Build history of the part. All positions in model axes, mm. Face numbers are marked on the shaded views. Give positions to 0.01 mm unless a question says otherwise; leave off trailing zeros. Write each loop counter-clockwise with the first axis right and the second up, starting at its lowest first coordinate (ties: lowest second). Pieces come first, ordered by that corner, then holes. Notation, with made-up numbers: (-15.75, 24.5) -> (-7.75, 24.5) arc R23 ccw to (-7.75, 45.5) -> close; hole circle Ø7 at (-4.75, 19). An arc over 180 degrees is marked (long way). Put each result on its own line as item: value. Start each with the question number.
Item 1: Slice it at A-A, the plane y = 0. List the corners of the cut face in (x, z), plus the area to 3 significant figures.
Item 2: Flat gauge pins, fed straight in: pin 1 Ø6 at (x, y) = (14.5, 7.5) entering from -Z; pin 2 Ø6 at (x, y) = (31, 19.5) entering from +Z; pin 3 Ø3 at (x, z) = (26, 6) entering from +Y. Where does each tip first touch, or does it go through?
Item 3: Drill centre lines: line 1 along X through (y, z) = (30.75, 0); line 2 along Z through (x, y) = (12.75, 0); line 3 along Z through (x, y) = (38, -16). Where is each one in solid material? Low to high.
Item 4: Two-plate mould, pull along Y, no slides. Class the marked faces 1, 2 and 3: pulls with the +Y half, pulls with the -Y half, needs draft (parallel to the pull), parting line crosses it, or undercut.
Item 5: Slice it at D-D, the plane x = 16. List the corners of the cut face in (y, z), plus the area to 3 significant figures.
Item 6: Slice it at C-C, the plane z = 0. Give the number of separate pieces and of enclosed holes in the cut face, plus the area to 3 significant figures.
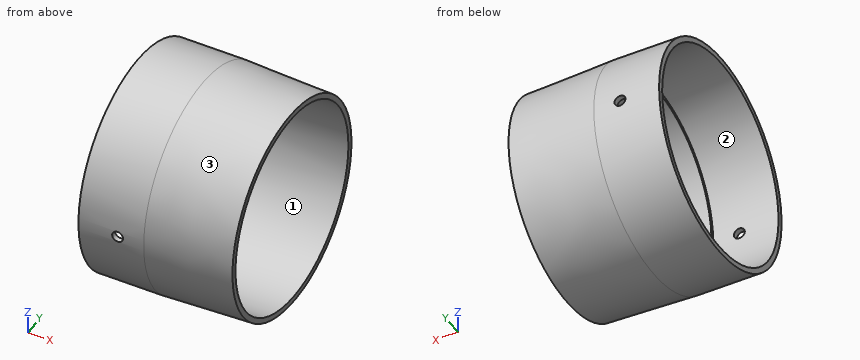
```python
from build123d import *

# Parameters (mm, degrees)
F0_R           = 31.8135
F1_DEPTH       = 19.05
F1_FACE_R      = 31.8135
F3_R           = 30.9245
F5_R           = 30.226
F6_DEPTH       = 19.05
F7_R           = 29.337
F8_DEPTH       = 25.4
F9_R           = 1.5875
F10_DEPTH      = 31.8145001
F10_DEPTH_BACK = 31.8145001


with BuildPart() as f1:
    # F0 (on Right) → F1 (new body)
    with BuildSketch(Plane.YZ):
        Circle(F0_R)
    extrude(amount=F1_DEPTH)

    # F1_face (on face) → F4 section 0
    with BuildSketch(Plane.YZ.offset(19.05)):
        Circle(F1_FACE_R)
    # F3 (on offset) → F4 section 1
    with BuildSketch(Plane.YZ.offset(44.45)):
        Circle(F3_R)
    loft()

    # F5 (on face) → F6 (cut)
    with BuildSketch(Plane(origin=(0, 0, 0), x_dir=(0, -1, 0), z_dir=(-1, 0, 0))):
        Circle(F5_R)
    extrude(amount=-F6_DEPTH, mode=Mode.SUBTRACT)

    # F7 (on face) → F8 (cut, through all)
    with BuildSketch(Plane.YZ.offset(44.45)):
        Circle(F7_R)
    extrude(amount=-F8_DEPTH, mode=Mode.SUBTRACT)

    # F9 (on Front) → F10 (cut, two sides)
    with BuildSketch(Plane.XZ) as f10_sk:
        with Locations((11.429999955, 0)):
            Circle(F9_R)
    extrude(amount=-F10_DEPTH, mode=Mode.SUBTRACT)
    extrude(f10_sk.sketch, amount=F10_DEPTH_BACK, mode=Mode.SUBTRACT)


solid = f1.part
```
Values follow:
1. outline: (0, -31.81) -> (19.05, -31.81) -> (44.45, -30.92) -> (44.45, -29.34) -> (19.05, -29.34) -> (19.05, -30.23) -> (0, -30.23) -> close; (0, 30.23) -> (19.05, 30.23) -> (19.05, 29.34) -> (44.45, 29.34) -> (44.45, 30.92) -> (19.05, 31.81) -> (0, 31.81) -> close
1. area: 164 mm2
2. pin 1: z = -31.49
2. pin 2: z = 26.71
2. pin 3: y = 31.25
3. line 1: 0 to 9.84, 13.02 to 44.45
3. line 2: -31.81 to -30.23, 30.23 to 31.81
3. line 3: -26.73 to -24.59, 24.59 to 26.73
4. face 1: undercut
4. face 2: undercut
4. face 3: parting line crosses it
5. outline: circle Ø63.63 at (0, 0); hole circle Ø60.45 at (0, 0)
5. area: 309 mm2
6. separate pieces: 4
6. enclosed holes: 0
6. area: 154 mm2
